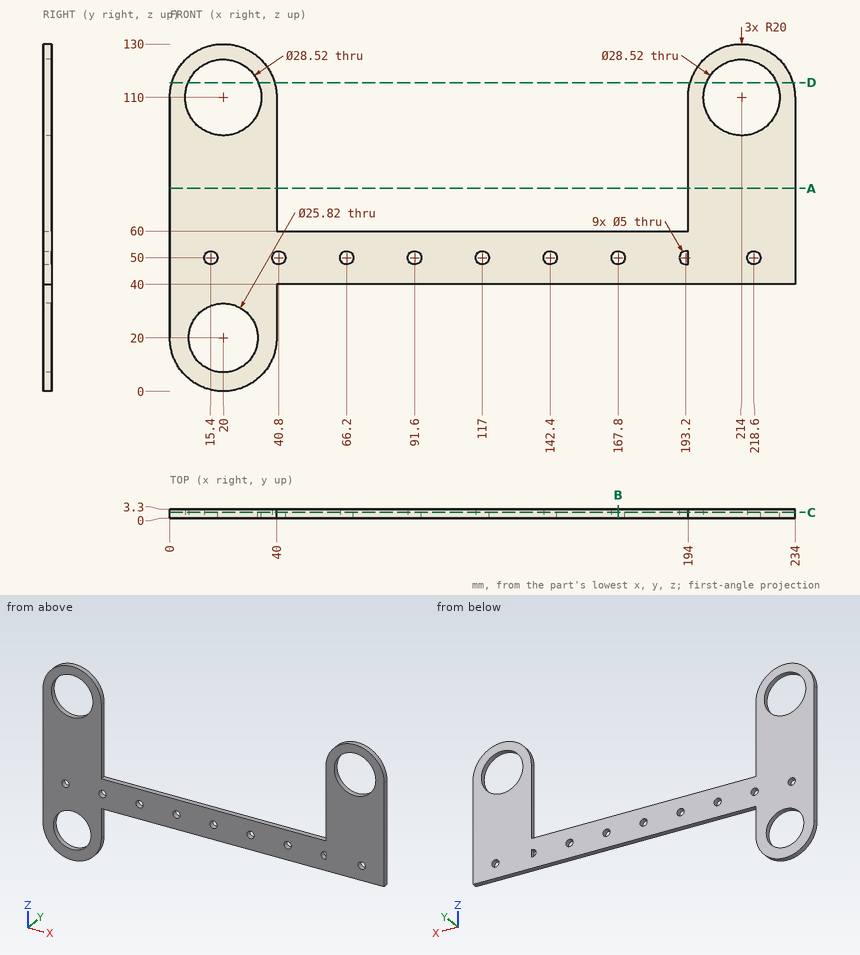
Design review of the part shown in the three views and the two pictorial views. Dimensions are in mm from the part's minimum x, y and z. Round coordinates to 2 decimals unless told otherwise and drop trailing zeros. Loops run counter-clockwise (first coordinate to the right, second up) from the corner with the lowest first, then second, coordinate; pieces in that order, holes last. Notation, with made-up numbers: (42.25, -17) - (61.25, -17) arc R30 cw to (61.25, 21) - close; hole circle Ø4 at (36, -24). An arc over 180 degrees is marked (long way). Use one line per item in the form item = value.
1) We need section A-A on z = 76. Write out the cut boundary in (x, y).
Solutions:
outline = (0, 0) - (40, 0) - (40, 3.3) - (0, 3.3) - close; (194, 0) - (234, 0) - (234, 3.3) - (194, 3.3) - close
2) Wall thickness on probe 1 along Z at (x, y) = (20, 1.05); probe 2 along Z at (x, y) = (142, 0.55); probe 3 along X at (y, z) = (1.85, 109.5): over which ranges is each line inside the solid? List them lowest first.
Solutions:
probe_1 = 0 to 7.09, 32.91 to 95.74, 124.26 to 130
probe_2 = 40 to 47.53, 52.47 to 60
probe_3 = 0 to 5.75, 34.25 to 40, 194 to 199.75, 228.25 to 234
3) Clearance check with flat-ended pins moving along their axes: P1, Ø6.5, axis at x = 218.6, z = 50, coming from the -Y side; P2, Ø4.5, axis at x = 66.2, z = 50, coming from the -Y side; P3, Ø1.5, axis at y = 2.5, z = 18.5, coming from the -X side; P4, Ø1.6, axis at x = 144.5, y = 2, coming from the -Z side. State where each tip first meets the part, or that it passes through.
Solutions:
P1 = 0
P2 = through
P3 = 0.01
P4 = 40
4) We need section C-C on y = 2.2. State how many separate pieces and enclosed holes the cut face has, then the cut area to 3 significant figures.
Solutions:
separate_pieces = 1
enclosed_holes = 12
area = 9,390 mm2
5) We need section B-B on x = 167.8. Write out the cut boundary in (y, z), then the cut area to 3 significant figures.
Solutions:
outline = (0, 40) - (3.3, 40) - (3.3, 47.5) - (0, 47.5) - close; (0, 52.5) - (3.3, 52.5) - (3.3, 60) - (0, 60) - close
area = 49.5 mm2
6) We need section D-D on z = 115.5. Write out the cut boundary in (x, y), then the cut area to 3 significant figures.
Solutions:
outline = (0.77, 0) - (6.84, 0) - (6.84, 3.3) - (0.77, 3.3) - close; (33.16, 0) - (39.23, 0) - (39.23, 3.3) - (33.16, 3.3) - close; (194.77, 0) - (200.84, 0) - (200.84, 3.3) - (194.77, 3.3) - close; (227.16, 0) - (233.23, 0) - (233.23, 3.3) - (227.16, 3.3) - close
area = 80.2 mm2
